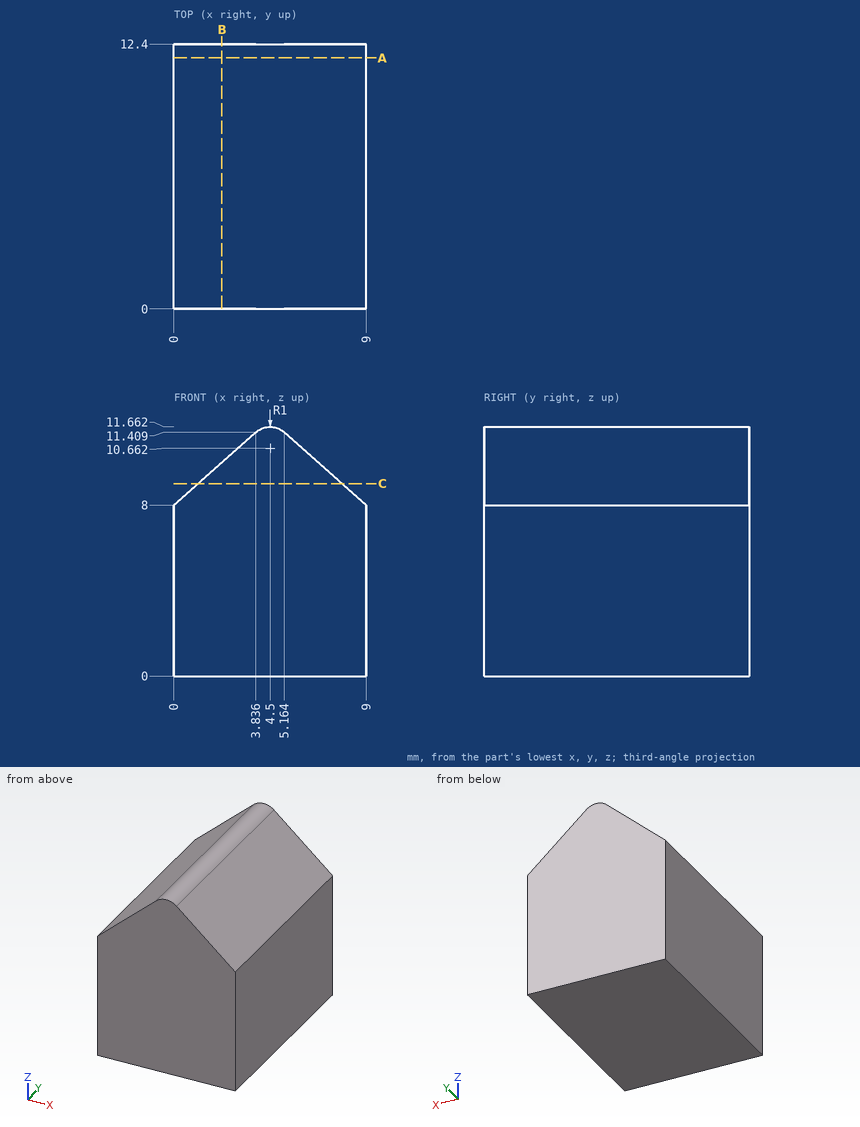
Could you check a few things on this drawing? It's one solid part, dimensions in mm from its lowest x, y, z. Round coordinates to 2 decimals unless told otherwise and drop trailing zeros. Write each loop counter-clockwise with the first axis right and the second up, starting at its lowest first coordinate (ties: lowest second). Pieces come first, ordered by that corner, then holes. Notation, with made-up numbers: (-31.5, 8.5) -> (-3.5, 8.5) arc R19 ccw to (-3.5, 31.5) -> close; hole circle Ø6 at (47, 30.25). An arc over 180 degrees is marked (long way). One line per question, with ' | ' between items. Start each with the question number.
1) Suppose I cut it at A-A on y = 11.75. Write out the boundary of the cut face in (x, z) (1 decimal).
2) Suppose I cut it at B-B on x = 2.25. Write out the boundary of the cut face in (y, z).
3) I need wall thicknesses on line 1 (X direction, y = 10.75, z = 9.5) (1 decimal); line 2 (Z direction, x = 2.5, y = 1.75); line 3 (Z direction, x = 2, y = 9). Which ranges of each line are inside material? Lowest first, please. Write a range as [from, to].
4) I'm going to push flat-ended pins straight in: P1, Ø3, axis at x = 5.5, y = 8, coming from the -Z side; P2, Ø1.5, axis at x = 5.5, y = 4.5, coming from the +Z side; P3, Ø1, axis at x = 7.5, y = 11, coming from the +Z side. Where does each tip first touch, or does it pass through?
5) Suppose I cut it at C-C on z = 9. Write out the boundary of the cut face in (x, y) (1 decimal).
Return value:
1) outline: (0, 0) -> (9, 0) -> (9, 8) -> (5.2, 11.4) arc R1 ccw to (3.8, 11.4) -> (0, 8) -> close
2) outline: (0, 0) -> (12.4, 0) -> (12.4, 10) -> (0, 10) -> close
3) line 1: x = [1.7, 7.3] | line 2: z = [0, 10.22] | line 3: z = [0, 9.78]
4) P1: stops at z = 0 | P2: stops at z = 11.63 | P3: stops at z = 9.78
5) outline: (1.1, 0) -> (7.9, 0) -> (7.9, 12.4) -> (1.1, 12.4) -> close
